Part print with two shaded views. Sizes in mm from the minimum x, y, z corner. A direction names the side the tool comes from. Round coordinates to 2 decimals unless told otherwise and drop trailing zeros. Write each loop counter-clockwise with the first axis right and the second up, starting at its lowest first coordinate (ties: lowest second). Pieces come first, ordered by that corner, then holes. Notation, with made-up numbers: (43, 57.25) -> (71, 57.25) arc R10 cw to (71, 74.25) -> close; hole circle Ø7 at (24, 11). An arc over 180 degrees is marked (long way). Answer as CSV lines item,"result".
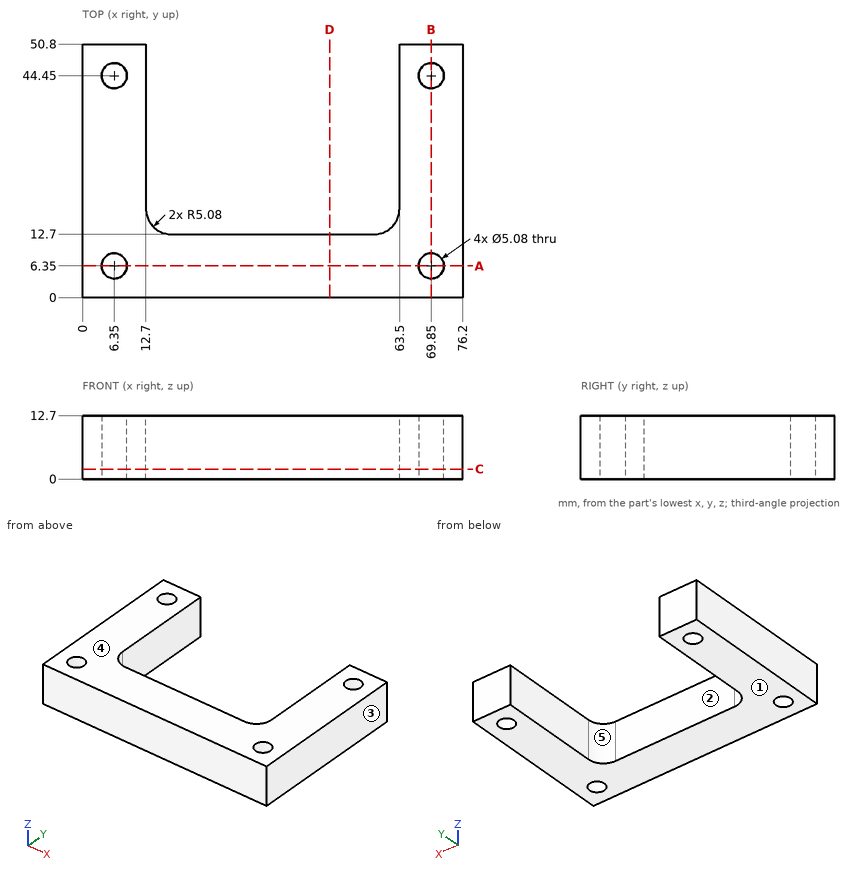
1. Probe line 1 along Y through (x, z) = (69.85, 2.5); line 2 along X through (y, z) = (6.35, 9.25); line 3 along X through (y, z) = (37.5, 10.75). List the from-to ranges inside material, lowest first.
Results found:
line 1,"y = 0 to 3.81, 8.89 to 41.91, 46.99 to 50.8"
line 2,"x = 0 to 3.81, 8.89 to 67.31, 72.39 to 76.2"
line 3,"x = 0 to 12.7, 63.5 to 76.2"
2. Cut at A-A, the plane y = 6.35. Write the cut outline in (x, z).
Results found:
outline,"(0, 0) -> (3.81, 0) -> (3.81, 12.7) -> (0, 12.7) -> close; (8.89, 0) -> (67.31, 0) -> (67.31, 12.7) -> (8.89, 12.7) -> close; (72.39, 0) -> (76.2, 0) -> (76.2, 12.7) -> (72.39, 12.7) -> close"
3. Cut at B-B, the plane x = 69.85. Write the cut outline in (y, z).
Results found:
outline,"(0, 0) -> (3.81, 0) -> (3.81, 12.7) -> (0, 12.7) -> close; (8.89, 0) -> (41.91, 0) -> (41.91, 12.7) -> (8.89, 12.7) -> close; (46.99, 0) -> (50.8, 0) -> (50.8, 12.7) -> (46.99, 12.7) -> close"
4. Cut at D-D, the plane x = 49.5. Write the cut outline in (y, z).
Results found:
outline,"(0, 0) -> (12.7, 0) -> (12.7, 12.7) -> (0, 12.7) -> close"
5. Drop flat-ended pins along their axis: pin 1 Ø6.5 at (x, y) = (69.85, 44.45) entering from -Z; pin 2 Ø5 at (x, z) = (30.5, 4.5) entering from +Y. Give the stop position or say it passes through.
Results found:
pin 1,"stops at z = 0"
pin 2,"stops at y = 12.7"
6. Which spindle directions (+Z, -Z, +X, -X, +Y, -Y) get a long thin tool onto all of the face, cutting with end or side? Do the marked faces 4 and 5. Say none if no direction does.
Results found:
face 4,"+Z, +X, -X, +Y, -Y"
face 5,"+Z, -Z, +Y"
7. Mould opens along X. For the marked faces 1, 2 and 3 say: +X half, -X half, draft (parallel to the pull), parting line (faces both ways), or undercut.
Results found:
face 1,"draft"
face 2,"undercut"
face 3,"+X half"
8. Cut at C-C, the plane z = 2. Write the cut outline in (x, y).
Results found:
outline,"(0, 0) -> (76.2, 0) -> (76.2, 50.8) -> (63.5, 50.8) -> (63.5, 17.78) arc R5.08 cw to (58.42, 12.7) -> (17.78, 12.7) arc R5.08 cw to (12.7, 17.78) -> (12.7, 50.8) -> (0, 50.8) -> close; hole circle Ø5.08 at (6.35, 6.35); hole circle Ø5.08 at (6.35, 44.45); hole circle Ø5.08 at (69.85, 6.35); hole circle Ø5.08 at (69.85, 44.45)"
